```python
from build123d import *

# Parameters (mm, degrees)
SKETCH1_R           = 1.6
SKETCH1_R_2         = 1.1
SKETCH1_R_3         = 2.1
SKETCH1_R_4         = 11
SKETCH1_W           = 32
SKETCH1_H           = 4
SKETCH1_W_2         = 20
SKETCH1_H_2         = 10
SKETCH1_W_3         = 41
SKETCH1_H_3         = 21
SKETCH1_W_4         = 5
BOSS_EXTRUDE1_DEPTH = 3
FILLET1_R           = 5


with BuildPart() as part:
    # Sketch1 → Boss-Extrude1 (new body)
    with BuildSketch(Plane(origin=(0, 0, 0), x_dir=(1, 0, 0), z_dir=(0, 1, 0))):
        with BuildLine():
            Line((-126.554445662, 87.5), (-104.054445662, 87.5))
            Line((-104.054445662, 87.5), (-18.218162556, 87.5))
            Line((-18.218162556, 87.5), (40.836283106, 87.5))
            Line((40.836283106, 87.5), (120.836283106, 87.5))
            Line((120.836283106, 87.5), (137.792290187, 87.5))
            Line((137.792290187, 87.5), (145.014445662, 87.5))
            ThreePointArc((145.014445662, 87.5), (168.46, 0), (145.014445662, -87.5))
            Line((145.014445662, -87.5), (137.792290187, -87.5))
            Line((137.792290187, -87.5), (120.836283106, -87.5))
            Line((120.836283106, -87.5), (40.836283106, -87.5))
            Line((40.836283106, -87.5), (-18.218162556, -87.5))
            Line((-18.218162556, -87.5), (-104.054445662, -87.5))
            Line((-104.054445662, -87.5), (-126.554445662, -87.5))
            ThreePointArc((-126.554445662, -87.5), (-150, 0), (-126.554445662, 87.5))
        make_face()
        with Locations((-110.77, 40)):
            Circle(SKETCH1_R, mode=Mode.SUBTRACT)
        with Locations((-110.77, -40)):
            Circle(SKETCH1_R, mode=Mode.SUBTRACT)
        with Locations((-125, -30)):
            Circle(SKETCH1_R, mode=Mode.SUBTRACT)
        with Locations((9.23, -36)):
            Circle(SKETCH1_R, mode=Mode.SUBTRACT)
        with Locations((143.46, -30)):
            Circle(SKETCH1_R, mode=Mode.SUBTRACT)
        with Locations((143.46, 30)):
            Circle(SKETCH1_R, mode=Mode.SUBTRACT)
        with Locations((9.23, 36)):
            Circle(SKETCH1_R, mode=Mode.SUBTRACT)
        with Locations((-125, 30)):
            Circle(SKETCH1_R, mode=Mode.SUBTRACT)
        with Locations((-137.5, 37)):
            Circle(SKETCH1_R_2, mode=Mode.SUBTRACT)
        with Locations((-137.5, 46.2)):
            Circle(SKETCH1_R_2, mode=Mode.SUBTRACT)
        with Locations((-137.5, -37)):
            Circle(SKETCH1_R_2, mode=Mode.SUBTRACT)
        with Locations((-137.5, -46.2)):
            Circle(SKETCH1_R_2, mode=Mode.SUBTRACT)
        with Locations((65.39, -77.245)):
            Circle(SKETCH1_R_3, mode=Mode.SUBTRACT)
        with Locations((65.39, -67.395)):
            Circle(SKETCH1_R_3, mode=Mode.SUBTRACT)
        with Locations((114.812291, -77.245)):
            Circle(SKETCH1_R_3, mode=Mode.SUBTRACT)
        with Locations((114.812291, -67.395)):
            Circle(SKETCH1_R_3, mode=Mode.SUBTRACT)
        with Locations((114.812291, 67.395)):
            Circle(SKETCH1_R_3, mode=Mode.SUBTRACT)
        with Locations((114.812291, 77.245)):
            Circle(SKETCH1_R_3, mode=Mode.SUBTRACT)
        with Locations((65.39, 67.395)):
            Circle(SKETCH1_R_3, mode=Mode.SUBTRACT)
        with Locations((65.39, 77.245)):
            Circle(SKETCH1_R_3, mode=Mode.SUBTRACT)
        with Locations((155.96, 37)):
            Circle(SKETCH1_R_2, mode=Mode.SUBTRACT)
        with Locations((155.96, 46.2)):
            Circle(SKETCH1_R_2, mode=Mode.SUBTRACT)
        with Locations((155.96, -46.2)):
            Circle(SKETCH1_R_2, mode=Mode.SUBTRACT)
        with Locations((155.96, -37)):
            Circle(SKETCH1_R_2, mode=Mode.SUBTRACT)
        with Locations((-46.927011093, -67.395)):
            Circle(SKETCH1_R_3, mode=Mode.SUBTRACT)
        with Locations((-46.927011093, -77.245)):
            Circle(SKETCH1_R_3, mode=Mode.SUBTRACT)
        with Locations((-96.349302093, -67.395)):
            Circle(SKETCH1_R_3, mode=Mode.SUBTRACT)
        with Locations((-96.349302093, -77.245)):
            Circle(SKETCH1_R_3, mode=Mode.SUBTRACT)
        with Locations((-96.349302093, 77.245)):
            Circle(SKETCH1_R_3, mode=Mode.SUBTRACT)
        with Locations((-96.349302093, 67.395)):
            Circle(SKETCH1_R_3, mode=Mode.SUBTRACT)
        with Locations((-46.927011093, 77.245)):
            Circle(SKETCH1_R_3, mode=Mode.SUBTRACT)
        with Locations((-46.927011093, 67.395)):
            Circle(SKETCH1_R_3, mode=Mode.SUBTRACT)
        with Locations((129.23, 40)):
            Circle(SKETCH1_R, mode=Mode.SUBTRACT)
        with Locations((129.23, -40)):
            Circle(SKETCH1_R, mode=Mode.SUBTRACT)
        with Locations((81.75, 26.5)):
            Circle(SKETCH1_R, mode=Mode.SUBTRACT)
        with Locations((146.828017544, 0)):
            Circle(SKETCH1_R_4, mode=Mode.SUBTRACT)
        with Locations((118.25, 26.5)):
            Circle(SKETCH1_R, mode=Mode.SUBTRACT)
        with Locations((81.75, -26.5)):
            Circle(SKETCH1_R, mode=Mode.SUBTRACT)
        with Locations((118.25, -26.5)):
            Circle(SKETCH1_R, mode=Mode.SUBTRACT)
        with Locations((9.23, 24)):
            Rectangle(SKETCH1_W, SKETCH1_H, mode=Mode.SUBTRACT)
        with Locations((9.23, -24)):
            Rectangle(SKETCH1_W, SKETCH1_H, mode=Mode.SUBTRACT)
        with Locations((9.23, 62.5)):
            Rectangle(SKETCH1_W_2, SKETCH1_H_2, mode=Mode.SUBTRACT)
        with Locations((9.23, -62.5)):
            Rectangle(SKETCH1_W_2, SKETCH1_H_2, mode=Mode.SUBTRACT)
        with Locations((90.1, 72.32)):
            Rectangle(SKETCH1_W_3, SKETCH1_H_3, mode=Mode.SUBTRACT)
        with Locations((90.1, -72.32)):
            Rectangle(SKETCH1_W_3, SKETCH1_H_3, mode=Mode.SUBTRACT)
        with Locations((-71.637011093, 72.32)):
            Rectangle(SKETCH1_W_3, SKETCH1_H_3, mode=Mode.SUBTRACT)
        with Locations((-71.637011093, -72.32)):
            Rectangle(SKETCH1_W_3, SKETCH1_H_3, mode=Mode.SUBTRACT)
        with Locations((-85, 40)):
            Rectangle(SKETCH1_W_4, SKETCH1_H_2, mode=Mode.SUBTRACT)
        with Locations((-85, -40)):
            Rectangle(SKETCH1_W_4, SKETCH1_H_2, mode=Mode.SUBTRACT)
        with Locations((103.46, 40)):
            Rectangle(SKETCH1_W_4, SKETCH1_H_2, mode=Mode.SUBTRACT)
        with Locations((103.46, -40)):
            Rectangle(SKETCH1_W_4, SKETCH1_H_2, mode=Mode.SUBTRACT)
    extrude(amount=BOSS_EXTRUDE1_DEPTH)

    # Fillet1
    fillet1_edges = [part.edges().sort_by_distance(p)[0] for p in [
        (-126.554445662, 1.5, 87.5),
        (-126.554445662, 1.5, -87.5),
        (145.014445662, 1.5, -87.5),
        (145.014445662, 1.5, 87.5),
    ]]
    fillet(fillet1_edges, radius=FILLET1_R)


solid = part.part
```
CAD build for the part. Positions are in the model's coordinates, mm. Give positions to 0.01 mm unless a question says otherwise; leave off trailing zeros. Loops run counter-clockwise (first coordinate to the right, second up) from the corner with the lowest first, then second, coordinate; pieces in that order, holes last. Notation, with made-up numbers: (60, 1) - (100, 1) arc R14 ccw to (100, 18) - close; hole circle Ø6 at (-3, 73.25). An arc over 180 degrees is marked (long way). Put each result on its own line as item: value.
Q1. Flat gauge pins, fed straight in: pin 1 (1 mm diameter, centred on y = 2.5, z = -58, fed in from -X); pin 2 (3 mm diameter, centred on x = 129.23, z = -40, fed in from +Y); pin 3 (1.5 mm diameter, centred on y = 1.5, z = 40.5, fed in from +X); pin 4 (1.5 mm diameter, centred on y = 1.5, z = -21, fed in from +X). Where does each tip first touch, or does it go through?
Filled in:
pin 1: stops at x = -140.28
pin 2: passes through
pin 3: stops at x = 163.89
pin 4: stops at x = 167.28
Q2. Slice it at A-A (z = 0). Give the cut face in (x, y), plus the area to 3 significant figures.
Filled in:
outline: (-150, 0) - (135.83, 0) - (135.83, 3) - (-150, 3) - close; (157.83, 0) - (168.46, 0) - (168.46, 3) - (157.83, 3) - close
area: 889 mm²
Q3. Mould opens along Z. For faces 1 (the face through (135.84, 1.48, -0.48)), 2 (the face through (-149.996, 1.479, 1.241)), 3 (the face through (11, 0, -1)) say: pulls with the +Z half, pulls with the -Z half, needs draft (parallel to the pull), parting line crosses it, or undercut.
Filled in:
face 1: undercut
face 2: parting line crosses it
face 3: needs draft
Q4. Probe line 1 along Z through (x, y) = (110.5, 0.5); line 2 along Z through (x, y) = (21, 2.2); line 3 along Z through (x, y) = (65.39, 1.5) (3 decimals). List the from-to ranges inside material, lowest first.
Filled in:
line 1: z = -87.5 to -82.82, -61.82 to 61.82, 82.82 to 87.5
line 2: z = -87.5 to -26, -22 to 22, 26 to 87.5
line 3: z = -87.5 to -79.345, -75.145 to -69.495, -65.295 to 65.295, 69.495 to 75.145, 79.345 to 87.5
Q5. Slice it at B-B (y = 1.75). Give the number of separate pieces and of enclosed holes in the cut face, plus the area to 3 significant figures.
Filled in:
separate pieces: 1
enclosed holes: 51
area: 48,000 mm²
